Model file for the job. Use its own axes, mm. Face numbers are marked on the shaded views. A direction names the side the tool comes from. Round coordinates to 2 decimals unless told otherwise and drop trailing zeros. Write each loop counter-clockwise with the first axis right and the second up, starting at its lowest first coordinate (ties: lowest second). Pieces come first, ordered by that corner, then holes.
```python
from build123d import *
from OCP.BRepAlgoAPI import BRepAlgoAPI_Cut
from OCP.TopTools import TopTools_ListOfShape

# Parameters (mm, degrees)
SKETCH1_R           = 4
SKETCH1_R_2         = 1.5
BOSS_EXTRUDE1_DEPTH = 6
SKETCH2_R           = 4
SKETCH2_R_2         = 3
BOSS_EXTRUDE2_DEPTH = 0.5
FILLET1_R           = 0.3
FILLET2_R           = 0.25
CIRPATTERN1_START   = -3
CIRPATTERN1_2_DEPTH = 3


with BuildPart() as part:
    # Sketch1 → Boss-Extrude1 (new body)
    with BuildSketch(Plane(origin=(0, 0, 0), x_dir=(1, 0, 0), z_dir=(0, 1, 0))):
        with Locations(Location((0, 0, 0), (0, 0, 270))):
            Circle(SKETCH1_R)
        with Locations(Location((0, 0, 0), (0, 0, 270))):
            Circle(SKETCH1_R_2, mode=Mode.SUBTRACT)
    extrude(amount=BOSS_EXTRUDE1_DEPTH)

    # Sketch2 → Boss-Extrude2 (add)
    with BuildSketch(Plane(origin=(0, 6, 0), x_dir=(1, 0, 0), z_dir=(0, 1, 0))):
        with Locations(Location((0, 0, 0), (0, 0, 270))):
            Circle(SKETCH2_R)
        with Locations(Location((0, 0, 0), (0, 0, 270))):
            Circle(SKETCH2_R_2, mode=Mode.SUBTRACT)
    extrude(amount=BOSS_EXTRUDE2_DEPTH)

    # Fillet1
    fillet1_edges = [part.edges().sort_by_distance(p)[0] for p in [
        (0, 6.5, -4),
        (0, 6.5, -3),
    ]]
    fillet(fillet1_edges, radius=FILLET1_R)

    # Fillet2
    fillet2_edges = [part.edges().sort_by_distance(p)[0] for p in [
        (0, 0, -4),
    ]]
    fillet(fillet2_edges, radius=FILLET2_R)


with BuildPart() as m4_tapped_hole1_tool:
    # M4 Tapped Hole1: read off the stored shape, not the designer's step
    # M4 Tapped Hole1 outline → M4 Tapped Hole1 (revolve)
    with BuildSketch(Plane.XZ.offset(-3)):
        Polygon((2.024995394, 3.999995394), (0, 3.999995394), (0, 0), (1.65, 0), (1.65, 3.625), align=None)
    revolve(axis=Axis((0, 3, 0), (0, 0, 1)))


with BuildPart() as part_1:
    add(part.part)

    # M4 Tapped Hole1: cut by m4_tapped_hole1_tool, with a tolerance
    m4_tapped_hole1_stock = TopTools_ListOfShape()
    m4_tapped_hole1_stock.Append(part_1.part.wrapped)
    m4_tapped_hole1_tools = TopTools_ListOfShape()
    m4_tapped_hole1_tools.Append(m4_tapped_hole1_tool.part.wrapped)
    m4_tapped_hole1_cut = BRepAlgoAPI_Cut()
    m4_tapped_hole1_cut.SetArguments(m4_tapped_hole1_stock)
    m4_tapped_hole1_cut.SetTools(m4_tapped_hole1_tools)
    m4_tapped_hole1_cut.SetFuzzyValue(0.00001)
    m4_tapped_hole1_cut.Build()
    add(Compound.cast(m4_tapped_hole1_cut.Shape()).solids(), mode=Mode.REPLACE)

    # CirPattern1: read off the stored shape, not the designer's step
    # CirPattern1 outline → CirPattern1 (revolve, cut)
    with BuildSketch(Plane(origin=(0, 3, 0), x_dir=(0, 1, 0), z_dir=(0, 0, -1))):
        Polygon((0, -4.000116403), (2.025116403, -4.000116403), (1.65, -3.625), (1.65, -1.575), (0, -1.575), align=None)
    revolve(axis=Axis((0, 3, 0), (1, 0, 0)), mode=Mode.SUBTRACT)

    # CirPattern1 2 outline → CirPattern1 2 (add)
    with BuildSketch(Plane.XY.offset(CIRPATTERN1_START)):
        with BuildLine():
            Line((-1.575, 2.508192111), (-1.575, 3.491807889))
            ThreePointArc((-1.575, 3.491807889), (-1.65, 3), (-1.575, 2.508192111))
        make_face()
    extrude(amount=CIRPATTERN1_2_DEPTH)


solid = part_1.part
```
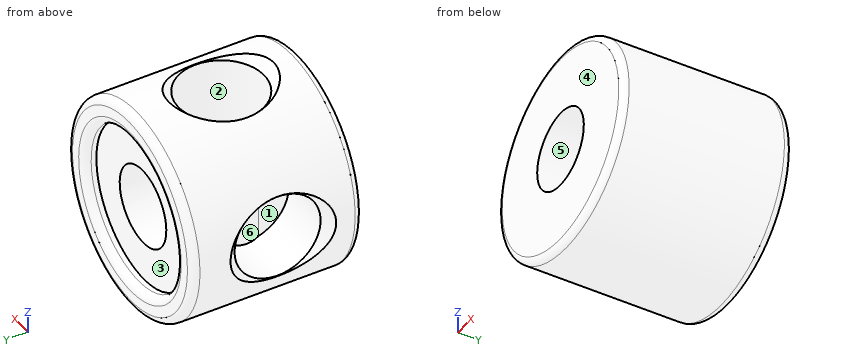
1) Cut at B-B on y = 3. List the corners of the cut face in (x, z) (3 decimals), and give its area (3 significant figures).
2) Flat gauge pins, fed straight in: pin 1 Ø0.9 at (y, z) = (2, 0) entering from -X (3 decimals); pin 2 Ø3 at (y, z) = (3.5, -2.5) entering from +X; pin 3 Ø3 at (x, z) = (-1, 0.5) entering from +Y. Where does each tip first touch, or does it go through?
3) Pull direction Y, two halves, no side cores. Call the marked faces 1, 2, 3 and 4: released by +Y, released by -Y, zero draft, split by the parting line, or undercut.
4) Which spindle directions (+Z, -Z, +X, -X, +Y, -Y) get a long thin tool onto all of the face, cutting with end or side? Do the marked faces 5 and 6. Say none if no direction does.
5) Wall check: probe 1 along Y at (x, z) = (-2.4, 0); probe 2 along Y at (x, z) = (1.5, 3); probe 3 along X at (y, z) = (6.1, 0). Give the ranges that are in metal, low to high.
6) Cut at A-A on x = 0. List the corners of the cut face in (y, z) (3 decimals), and give its area (3 significant figures).
7) Cut at C-C on z = 1. Give the number of separate pieces and of enclosed holes in the cut face, and give its area (3 significant figures).
Result sheet:
1. outline: (-3.638, -1.663) arc R4 ccw (long way) to (1.663, 3.638) - (1.65, 3.625) - (1.65, 0) - (1.5, 0) arc R1.5 cw to (-1.5, 0) - (-1.65, 0) - (-1.65, -1.65) - (-3.625, -1.65) - close; (-3.638, 1.663) - (-3.625, 1.65) - (-1.65, 1.65) - (-1.65, 3.625) - (-1.663, 3.638) arc R4 ccw to start
1. area: 26.5 mm2
2. pin 1: stops at x = -1.575
2. pin 2: stops at x = 3.87
2. pin 3: stops at y = 6
3. face 1: undercut
3. face 2: undercut
3. face 3: released by +Y
3. face 4: released by -Y
4. face 5: +Y, -Y
4. face 6: -X
5. probe 1: y = 0 to 1.35, 4.65 to 6
5. probe 2: y = 0 to 2.31, 3.69 to 6.5
5. probe 3: x = -4 to -3, 3 to 4
6. outline: (0, -3.75) arc R0.25 ccw to (0.25, -4) - (6.2, -4) arc R0.3 ccw to (6.5, -3.7) - (6.5, -3.3) arc R0.3 ccw to (6.2, -3) - (6, -3) - (6, -1.5) - (0, -1.5) - close; (0, 1.5) - (1.35, 1.5) - (1.35, 3.625) - (0.975, 4) - (0.25, 4) arc R0.25 ccw to (0, 3.75) - close; (4.65, 1.5) - (6, 1.5) - (6, 3) - (6.2, 3) arc R0.3 ccw to (6.5, 3.3) - (6.5, 3.7) arc R0.3 ccw to (6.2, 4) - (5.025, 4) - (4.65, 3.625) - close
6. area: 22.5 mm2
7. separate pieces: 3
7. enclosed holes: 0
7. area: 26.2 mm2
